Design review of the part shown in the three views and the two pictorial views. Dimensions are in mm from the part's minimum x, y and z. Round coordinates to 2 decimals unless told otherwise and drop trailing zeros. Loops run counter-clockwise (first coordinate to the right, second up) from the corner with the lowest first, then second, coordinate; pieces in that order, holes last.
1) Take a section at C-C (x = 10). State the section outline as (y, z) points (1 decimal).
2) Insertion check: pin 1 (3 mm diameter, centred on y = 17, z = 35.5, fed in from +X); pin 2 (2 mm diameter, centred on y = 8.5, z = 23, fed in from +X); pin 3 (5 mm diameter, centred on y = 24, z = 18, fed in from -X). Each pin has a flat end and moves straight along its axis. Give the tip position at first contact, or say it passes through.
3) Wall thickness on L1, parallel to X at y = 9, z = 13.5 (1 decimal); L2, parallel to X at y = 8, z = 29 (1 decimal); L3, parallel to Z at x = 33, y = 22.75 (1 decimal): over which ranges is each line inside the solid? List them lowest first.
4) Take a section at A-A (y = 16.75). State the section outline as (x, z) points (1 decimal), then the cut area to 3 significant figures.
5) Take a section at D-D (x = 27). State the section outline as (y, z) points (1 decimal).
6) Take a section at B-B (z = 21). State the section outline as (x, y) points (1 decimal).
7) Mouldability with a two-part tool opening along Y and no side actions: class the marked faces 1, 2, 3 and 4 as pulls with the +Y half, pulls with the -Y half, needs draft (parallel to the pull), parting line crosses it, or undercut.
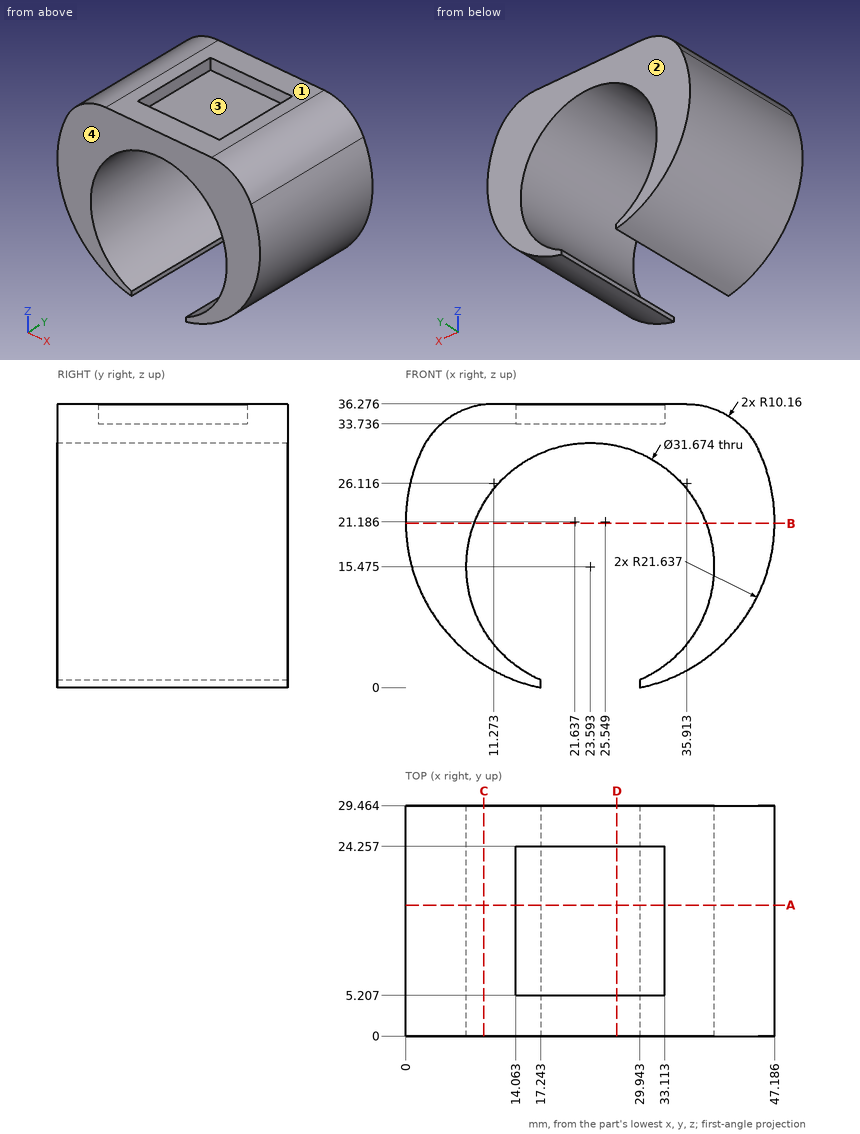
Response:
1. outline: (0, 2.9) - (29.5, 2.9) - (29.5, 7.3) - (0, 7.3) - close; (0, 23.6) - (29.5, 23.6) - (29.5, 36.2) - (0, 36.2) - close
2. pin 1: stops at x = 42.32
2. pin 2: stops at x = 47.17
2. pin 3: stops at x = 0.01
3. L1: x = 1.4 to 7.9, 39.3 to 45.8
3. L2: x = 1.5 to 15.4, 31.8 to 45.7
3. L3: z = 0.9 to 2.7, 28.2 to 33.7
4. outline: (2.1, 30.5) arc R21.6 ccw to (17.2, 0) - (17.2, 1) arc R15.8 cw (long way) to (29.9, 1) - (29.9, 0) arc R21.6 ccw to (45.1, 30.5) arc R10.2 ccw to (35.9, 36.3) - (33.1, 36.3) - (33.1, 33.7) - (14.1, 33.7) - (14.1, 36.3) - (11.3, 36.3) arc R10.2 ccw to start
4. area: 623 mm2
5. outline: (0, 30.9) - (29.5, 30.9) - (29.5, 36.3) - (24.3, 36.3) - (24.3, 33.7) - (5.2, 33.7) - (5.2, 36.3) - (0, 36.3) - close
6. outline: (0, 0) - (8.8, 0) - (8.8, 29.5) - (0, 29.5) - close; (38.4, 0) - (47.2, 0) - (47.2, 29.5) - (38.4, 29.5) - close
7. face 1: needs draft
7. face 2: pulls with the +Y half
7. face 3: undercut
7. face 4: pulls with the -Y half
